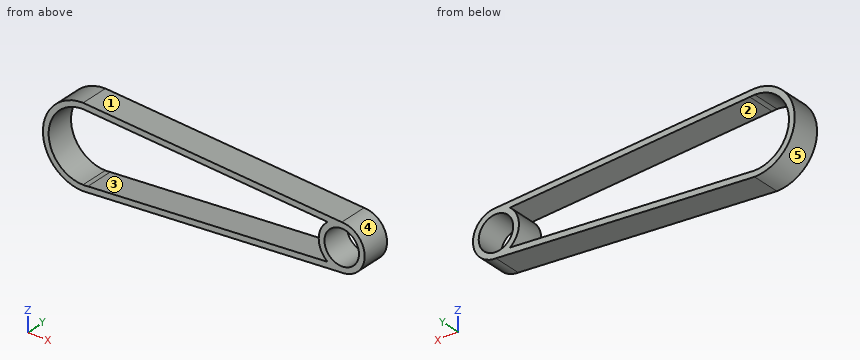
from build123d import *

# Parameters (mm, degrees)
SKETCH1_R           = 6
BOSS_EXTRUDE1_DEPTH = 10


with BuildPart() as part:
    # Sketch1 → Boss-Extrude1 (new body)
    with BuildSketch(Plane(origin=(0, 0, 0), x_dir=(1, 0, 0), z_dir=(0, 1, 0))):
        with BuildLine():
            ThreePointArc((0, 14), (-14, 0), (0, -14))
            Line((0, -14), (90, -8))
            ThreePointArc((90, -8), (98, 0), (90, 8))
            Line((90, 8), (0, 14))
        make_face()
        with BuildLine():
            ThreePointArc((1.65636135, -11.885136393), (0.798228126, -11.973421894), (-0.064030313, -11.99982917))
            ThreePointArc((-0.064030313, -11.99982917), (-12, 0), (-0.064030313, 11.99982917))
            ThreePointArc((-0.064030313, 11.99982917), (0.798228126, 11.973421894), (1.65636135, 11.885136393))
            Line((1.65636135, 11.885136393), (85.098173392, 6.322348923))
            ThreePointArc((85.098173392, 6.322348923), (82, 0), (85.098173392, -6.322348923))
            Line((85.098173392, -6.322348923), (1.65636135, -11.885136393))
        make_face(mode=Mode.SUBTRACT)
        with Locations((90, 0)):
            Circle(SKETCH1_R, mode=Mode.SUBTRACT)
    extrude(amount=BOSS_EXTRUDE1_DEPTH)


solid = part.part
Design review of the part built by this model. Coordinates are the model's own, in mm. Face numbers are marked on the shaded views. A direction names the side the tool comes from. Coordinates: 2 decimals unless noted, no trailing zeros. Order: outer loops, then holes, each group sorted by start corner. A loop starts at its lowest first (then second) coordinate and runs counter-clockwise, first axis right, second up.
Item 1: For the marked faces 1 and 2, list the 3-axis set-ups (+Z, -Z, +X, -X, +Y, -Y) from which the entire face can be reached by the end or side of a thin tool; tool diameter is ignored.
Item 2: Take a section at C-C, the plane x = -4. Write out the cut boundary in (y, z), then the cut area to 3 significant figures.
Item 3: Take a section at B-B, the plane y = 7.25. Write out the cut boundary in (x, z), then the cut area to 3 significant figures.
Item 4: Take a section at A-A, the plane z = 0. Write out the cut boundary in (x, y).
Item 5: The part is to be moulded in two halves that separate along X. For the marked faces 3, 4 and 5, say which applies: pulls with the +X half, pulls with the -X half, needs draft (parallel to the pull), parting line crosses it, or undercut.
Item 6: For pin 1 Ø1 at (x, y) = (83, 4.5) entering from -Z; pin 2 Ø2 at (x, z) = (52.5, -5.5) entering from -Y; pin 3 Ø2 at (x, y) = (37.5, 1.5) entering from -Z; pin 4 Ø1.5 at (x, y) = (16.5, 1.5) entering from +Z, all flat-tipped, find the tip position at first contact; note any pin that passes through.
Item 7: For line 1 (X direction, y = 3.75, z = 0); line 2 (Z direction, x = 90, y = 4.5); line 3 (X direction, y = 0.5, z = 1.5), list the stretches that pass through material, from the lowest coordinate up.
Item 8: Take a section at D-D, the plane z = -4.5. Write out the cut boundary in (x, y).
The answers:
1. face 1: +Z, +X, +Y, -Y
1. face 2: +Y, -Y
2. outline: (0, -13.42) - (10, -13.42) - (10, -11.31) - (0, -11.31) - close; (0, 11.31) - (10, 11.31) - (10, 13.42) - (0, 13.42) - close
2. area: 42.1 mm2
3. outline: (0, -14) - (90, -8) arc R8 ccw to (90, 8) - (0, 14) arc R14 ccw to start; hole (1.66, -11.89) - (85.1, -6.32) arc R8 cw to (85.1, 6.32) - (1.66, 11.89) arc R12 ccw (long way) to start; hole circle Ø12 at (90, 0)
3. area: 518 mm2
4. outline: (-14, 0) - (-12, 0) - (-12, 10) - (-14, 10) - close; (82, 0) - (84, 0) - (84, 10) - (82, 10) - close; (96, 0) - (98, 0) - (98, 10) - (96, 10) - close
5. face 3: undercut
5. face 4: pulls with the +X half
5. face 5: pulls with the -X half
6. pin 1: stops at z = -8.5
6. pin 2: passes through
6. pin 3: stops at z = -11.57
6. pin 4: stops at z = 12.95
7. line 1: x = -14 to -12, 82 to 84, 96 to 98
7. line 2: z = -8 to -6, 6 to 8
7. line 3: x = -13.92 to -11.91, 82.14 to 84.19, 95.81 to 97.86
8. outline: (-13.26, 0) - (-11.12, 0) - (-11.12, 10) - (-13.26, 10) - close; (83.39, 0) - (86.03, 0) - (86.03, 10) - (83.39, 10) - close; (93.97, 0) - (96.61, 0) - (96.61, 10) - (93.97, 10) - close
